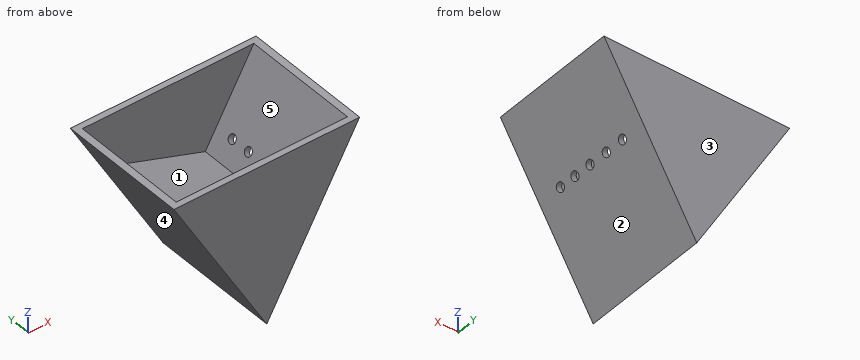
from build123d import *

# Parameters (mm, degrees)
F1_DEPTH = 105
F2_T     = -5
F4_DEPTH = 95
F6_D     = 7


with BuildPart() as f1:
    # F0 (on Front) → F1 (new body)
    with BuildSketch(Plane.XZ):
        Polygon((74.57273, 75.522542), (-75.42727, 75.522542), (-0.42727, -54.381269), align=None)
    extrude(amount=F1_DEPTH)

    # F2
    f2_openings = [f1.faces().sort_by_distance(p)[0] for p in [
        (-0.42727, -52.5, 75.522542),
    ]]
    offset(amount=F2_T, openings=f2_openings)

    # F3 (on face) → F4 (join)
    with BuildSketch(Plane.XZ.offset(5)):
        Polygon((29.57273, 7.580256), (-45.42727, 33.561018), (-0.42727, -44.381269), align=None)
    extrude(amount=F4_DEPTH)

    # F6 (through all)
    with Locations(Plane(origin=(18.897201, 0, -10.910304), x_dir=(0, -1, 0), z_dir=(-0.866025, 0, 0.5))):
        with Locations((83.523616, 39.900303), (20.983379, 39.36794), (37.380986, 39.312027), (53.739835, 39.52726), (68.919398, 39.673682)):
            Hole(F6_D / 2)


solid = f1.part
Read the model definition and answer for the solid it produces. Units are mm, in the model's axes. Face numbers are marked on the shaded views. A direction names the side the tool comes from. Coordinates: 2 decimals unless noted, no trailing zeros. Order: outer loops, then holes, each group sorted by start corner. A loop starts at its lowest first (then second) coordinate and runs counter-clockwise, first axis right, second up. Notation, with made-up numbers: M 39,2 L 62,2 A8 ccw 62,7 Z; hole C 28.5,67 d9. An arc over 180 degrees is marked long. Put each result on its own line as item: value. Start each with the question number.
Item 1: Section C-C, the plane y = -31.5 is taken. Determine the outline of the cut face in (x, z).
Item 2: For the marked faces 1 and 2, determine the directions among +Z, -Z, +X, -X, +Y, -Y from which every point of the face is accessible in a straight line to the end or side of a thin tool.
Item 3: The mould has two halves that part along Y. Classify the marked faces 3, 4 and 5: +Y half, -Y half, draft (parallel to the pull), parting line (faces both ways), or undercut.
Item 4: Consider probe 1 along Y at (x, z) = (-28, 53); probe 2 along X at (y, z) = (-67.5, 37.5); probe 3 along Z at (x, y) = (-14, -70.5). Determine where each line is inside the solid, lowest interval first. Write a range as [from, to].
Item 5: Section D-D, the plane x = 48 is taken. Determine the outline of the cut face in (y, z).
Item 6: Section A-A, the plane z = 54 is taken. Determine the outline of the cut face in (x, y), plus the area to 3 significant figures.
Item 7: Given pin 1 Ø12 at (x, y) = (-12.5, -62.5) entering from -Z; pin 2 Ø3 at (y, z) = (-20.5, 35.5) entering from -X; pin 3 Ø6 at (x, y) = (58, -56) entering from -Z, each flat-ended and moving along its own axis, determine where each tip first touches the part or whether it passes through.
Item 8: Section B-B, the plane y = -69 is taken. Determine the outline of the cut face in (x, z), plus the area to 3 significant figures.
Computed:
1. outline: M -75.43,75.52 L -0.43,-54.38 L 74.57,75.52 L 68.8,75.52 L 29.57,7.58 L -45.43,33.56 L -69.65,75.52 Z
2. face 1: +Z
2. face 2: -Z, +X, +Y, -Y
3. face 3: +Y half
3. face 4: draft
3. face 5: undercut
4. probe 1: y = [-105, -100], [-5, 0]
4. probe 2: x = [-53.47, -47.7], [46.85, 52.62]
4. probe 3: z = [-30.87, 22.67]
5. outline: M -105,29.5 L 0,29.5 L 0,75.52 L -5,75.52 L -5,39.5 L -100,39.5 L -100,75.52 L -105,75.52 Z
6. outline: M -63,-105 L 62.15,-105 L 62.15,0 L -63,0 Z; hole M -57.23,-100 L 56.37,-100 L 56.37,-5 L -57.23,-5 Z
6. area: 2,350 mm2
7. pin 1: stops at z = -43.86
7. pin 2: stops at x = -53.19
7. pin 3: stops at z = 41.62
8. outline: M -75.43,75.52 L -0.43,-54.38 L 41.31,17.92 L 36.98,20.42 L 29.57,7.58 L -45.43,33.56 L -69.65,75.52 Z; M 40.48,26.48 L 44.81,23.98 L 74.57,75.52 L 68.8,75.52 Z
8. area: 3,750 mm2
